Can you work these out from the model? Positions are in its coordinate system, mm. A direction names the side the tool comes from. Coordinates: 2 decimals unless noted, no trailing zeros. Write each loop counter-clockwise with the first axis right and the second up, starting at its lowest first coordinate (ties: lowest second). Pieces come first, ordered by that corner, then holes.
Autodesk Inventor part; units mm, degrees
ref_plane "YZ Plane" through (0, 0, 0) normal (1, 0, 0) x (0, 1, 0)
ref_plane "XZ Plane" through (0, 0, 0) normal (0, 1, 0) x (-1, 0, 0)
ref_plane "XY Plane" through (0, 0, 0) normal (0, 0, 1) x (1, 0, 0)
sketch "Sketch1" plane through (0, 0, 0) normal (0, 0, 1) x (1, 0, 0)
  line L0 (0, 0) -> (148, 0)
  line L1 (148, 0) -> (148, 210)
  line L2 (148, 210) -> (0, 210)
  line L3 (0, 210) -> (0, 0)
  dimension "d0" = 148
  dimension "d1" = 210
extrude "Extrusion1" add sketch "Sketch1" along normal blind 3
sketch "Sketch2" plane through (0, 0, 3) normal (0, 0, 1) x (1, 0, 0)
  line L0 (0, 0) -> (0, 210)
  line L1 (148, 0) -> (0, 0)
  line L2 (148, 210) -> (148, 0)
  line L3 (0, 210) -> (148, 210)
  line L4 (4, 185) -> (7, 185)
  line L5 (7, 185) -> (7, 175)
  line L6 (7, 175) -> (4, 175)
  line L7 (4, 175) -> (4, 185)
  line L8 (4, 40) -> (7, 40)
  line L9 (7, 40) -> (7, 30)
  line L10 (7, 30) -> (4, 30)
  line L11 (4, 30) -> (4, 40)
  line L12 (4, 20) -> (7, 20)
  line L13 (7, 20) -> (7, 10)
  line L14 (7, 10) -> (4, 10)
  line L15 (4, 10) -> (4, 20)
  line L16 (141, 185) -> (144, 185)
  line L17 (144, 185) -> (144, 175)
  line L18 (144, 175) -> (141, 175)
  line L19 (141, 175) -> (141, 185)
  line L20 (141, 40) -> (144, 40)
  line L21 (144, 40) -> (144, 30)
  line L22 (144, 30) -> (141, 30)
  line L23 (141, 30) -> (141, 40)
  line L24 (141, 20) -> (144, 20)
  line L25 (144, 20) -> (144, 10)
  line L26 (144, 10) -> (141, 10)
  line L27 (141, 10) -> (141, 20)
  dimension "d8" = 10
  dimension "d10" = 10
  dimension "d11" = 10
  dimension "d12" = 10
  dimension "d13" = 10
  dimension "d16" = 10
  dimension "d17" = 10
  dimension "d18" = 10
  dimension "d19" = 10
  dimension "d43" = 4
  dimension "d44" = 4
  dimension "d45" = 3
  dimension "d46" = 3
  dimension "d47" = 4
  dimension "d48" = 3
  dimension "d49" = 3
  dimension "d50" = 4
  dimension "d51" = 4
  dimension "d52" = 3
  dimension "d194" = 25
  dimension "d195" = 25
extrude "Extrusion2" cut sketch "Sketch2" against normal through all contours L4 L5 L6 L7 | L8 L9 L10 L11 | L12 L13 L14 L15 | L16 L17 L18 L19 | L20 L21 L22 L23 | L24 L25 L26 L27
sketch "Sketch3" plane through (0, 0, 3) normal (0, 0, 1) x (1, 0, 0)
  line L0 (7, 30) -> (4, 30)
  line L1 (7, 20) -> (7, 10)
  line L2 (0, 210) -> (148, 210)
  line L3 (7, 185) -> (7, 175)
  line L4 (141, 175) -> (141, 185)
  point P0 (5.5, 190)
  point P1 (142.5, 190)
  point P2 (5.5, 25)
  point P3 (142.5, 25)
  point P4 (141, 30)
  dimension "d24" = 5
  dimension "d54" = 1.5
  dimension "d189" = 1.5
  dimension "d192" = 20
  dimension "d193" = 20
  dimension "d196" = 1.5
  dimension "d197" = 1.5
hole "Hole1" at (5.5, 190, 3) at (142.5, 190, 3) at (5.5, 25, 3) at (142.5, 25, 3) direction (0, 0, -1) diameter 3 end through all
fillet "Fillet1" radius 2 4 edges at (0, 0, 1.5) (148, 0, 1.5) (0, 210, 1.5) (148, 210, 1.5)
sketch "Sketch4" plane through (0, 0, 3) normal (0, 0, 1) x (1, 0, 0)
  line L0 (7, 20) -> (7, 10)
  line L1 (141, 10) -> (141, 20)
  line L2 (146, 0) -> (2, 0)
  line L3 (17, 26.5) -> (27, 26.5)
  line L4 (27, 26.5) -> (27, 23.5)
  line L5 (27, 23.5) -> (17, 23.5)
  line L6 (17, 23.5) -> (17, 26.5)
  line L7 (121, 23.5) -> (131, 23.5)
  line L8 (131, 23.5) -> (131, 26.5)
  line L9 (131, 26.5) -> (121, 26.5)
  line L10 (121, 26.5) -> (121, 23.5)
  line L11 (2, 210) -> (146, 210)
  line L12 (17, 204.5) -> (27, 204.5)
  line L13 (27, 204.5) -> (27, 201.5)
  line L14 (27, 201.5) -> (17, 201.5)
  line L15 (17, 201.5) -> (17, 204.5)
  line L16 (121, 204.5) -> (131, 204.5)
  line L17 (131, 204.5) -> (131, 201.5)
  line L18 (131, 201.5) -> (121, 201.5)
  line L19 (121, 201.5) -> (121, 204.5)
  line L20 (69, 26.5) -> (79, 26.5)
  line L21 (79, 26.5) -> (79, 23.5)
  line L22 (79, 23.5) -> (69, 23.5)
  line L23 (69, 23.5) -> (69, 26.5)
  line L24 (69, 204.5) -> (79, 204.5)
  line L25 (79, 204.5) -> (79, 201.5)
  line L26 (79, 201.5) -> (69, 201.5)
  line L27 (69, 201.5) -> (69, 204.5)
  line L28 (7, 185) -> (7, 175)
  line L29 (141, 175) -> (141, 185)
  dimension "d33" = 10
  dimension "d34" = 23.5
  dimension "d35" = 3
  dimension "d36" = 10
  dimension "d37" = 3
  dimension "d39" = 10
  dimension "d40" = 10
  dimension "d82" = 10
  dimension "d83" = 3
  dimension "d84" = 5.5
  dimension "d85" = 10
  dimension "d86" = 42
  dimension "d89" = 10
  dimension "d90" = 10
  dimension "d91" = 42
  dimension "d92" = 5.5
  dimension "d93" = 3
  dimension "d198" = 10
  dimension "d199" = 10
extrude "Extrusion3" cut sketch "Sketch4" against normal through all
sketch "草圖15" plane through (0, 0, 3) normal (0, 0, 1) x (1, 0, 0)
  line L0 (0, 2) -> (0, 208)
  line L1 (146, 0) -> (2, 0)
  line L2 (148, 208) -> (148, 2)
  line L3 (95, 16.5) -> (105, 16.5)
  line L4 (108, 13.5) -> (108, 13.5)
  line L5 (105, 10.5) -> (95, 10.5)
  line L6 (92, 13.5) -> (92, 13.5)
  arc A0 (108, 13.5) -> (105, 16.5) centre (105, 13.5) ccw
  arc A1 (105, 10.5) -> (108, 13.5) centre (105, 13.5) ccw
  arc A2 (92, 13.5) -> (95, 10.5) centre (95, 13.5) ccw
  arc A3 (95, 16.5) -> (92, 13.5) centre (95, 13.5) ccw
  arc A4 (48.0314, 9) -> (48.0314, 18) centre (52, 13.5) ccw
  line L7 (38, 17.5) -> (46.7085, 17.5)
  line L8 (46.7085, 9.5) -> (38, 9.5)
  line L9 (34, 13.5) -> (34, 13.5)
  arc A5 (38, 17.5) -> (34, 13.5) centre (38, 13.5) ccw
  arc A6 (34, 13.5) -> (38, 9.5) centre (38, 13.5) ccw
  arc A7 (46.7085, 17.5) -> (48.0314, 18) centre (46.7085, 19.5) ccw
  arc A8 (48.0314, 9) -> (46.7085, 9.5) centre (46.7085, 7.5) ccw
  point P0 (0, 0)
  point P1 (92, 16.5)
  point P2 (108, 16.5)
  point P3 (92, 10.5)
  point P4 (34, 17.5)
  point P5 (34, 9.5)
  point P6 (47.5279, 17.5)
  point P7 (47.5279, 9.5)
  dimension "d159" = 16
  dimension "d161" = 6
  dimension "d163" = 40
  dimension "d164" = 3
  dimension "d165" = 12
  dimension "d166" = 13.5
  dimension "d167" = 13.5
  dimension "d168" = 52
  dimension "d169" = 8
  dimension "d173" = 4
  dimension "d174" = 2
extrude "擠出8" cut sketch "草圖15" against normal through all
sketch "草圖16" plane through (0, 0, 3) normal (0, 0, 1) x (1, 0, 0)
  line L0 (0, 2) -> (0, 208)
  line L1 (146, 0) -> (2, 0)
  point P0 (0, 0)
  point P1 (59, 32)
  point P2 (89, 32)
  point P3 (59, 62)
  point P4 (89, 62)
  dimension "d177" = 32
  dimension "d178" = 30
  dimension "d180" = 59
  dimension "d181" = 30
hole "孔7" at (59, 32, 3) at (89, 32, 3) at (59, 62, 3) at (89, 62, 3) direction (0, 0, -1) diameter 4 end through all
properties part number "plastic_part_1"
1. If we section it at B-B, the plane x = 75: List the corners of the cut face in (y, z) for me.
2. If we section it at C-C, the plane z = 1.2: Count the separate pieces of the cut face and the enclosed holes in it, plus the area to 3 significant figures.
3. We'd pull the mould along Y, two halves only. Please class faces 1 (the face through (57.314, 30.925, 1.479)), 2 (the face through (73, 106, 0)), 3 (the face through (87.314, 30.925, 1.479)): released by +Y, released by -Y, zero draft, split by the parting line, or undercut.
4. If we section it at A-A, the plane x = 52: List the corners of the cut face in (y, z) for me, plus the area to 3 significant figures.
5. If I drill on L1, parallel to Y at x = 122, z = 0.15; L2, parallel to Y at x = 5.5, z = 2.25; L3, parallel to X at y = 32, z = 1.3, over which ranges is the centre line in solid material (lowest first)?
6. Which directions (+Z, -Z, +X, -X, +Y, -Y) give clear straight access to the entire face, cutting with the end or side of a thin tool? Please do faces 4 (the face through (34, 13.6, 1.5)), 5 (the face through (73, 106, 3)).
Answers:
1. outline: (0, 0) - (23.5, 0) - (23.5, 3) - (0, 3) - close; (26.5, 0) - (201.5, 0) - (201.5, 3) - (26.5, 3) - close; (204.5, 0) - (210, 0) - (210, 3) - (204.5, 3) - close
2. separate pieces: 1
2. enclosed holes: 22
2. area: 30,300 mm2
3. face 1: undercut
3. face 2: zero draft
3. face 3: undercut
4. outline: (0, 0) - (7.5, 0) - (7.5, 3) - (0, 3) - close; (19.5, 0) - (210, 0) - (210, 3) - (19.5, 3) - close
4. area: 594 mm2
5. L1: y = 0 to 23.5, 26.5 to 201.5, 204.5 to 210
5. L2: y = 0 to 10, 20 to 23.5, 26.5 to 30, 40 to 175, 185 to 188.5, 191.5 to 210
5. L3: x = 0 to 4, 7 to 57, 61 to 87, 91 to 141, 144 to 148
6. face 4: +Z, -Z
6. face 5: +Z, +X, -X, +Y, -Y
